The listing builds one solid part. Answer for the finished solid, in the listing's coordinates (mm). A direction names the side the tool comes from. Give positions to 0.01 mm unless a question says otherwise; leave off trailing zeros. Write each loop counter-clockwise with the first axis right and the second up, starting at its lowest first coordinate (ties: lowest second). Pieces come first, ordered by that corner, then holes. Notation, with made-up numbers: (-32, 39.25) - (22, 39.25) arc R31 ccw to (22, 74.25) - close; hole circle Ø11 at (32.25, -22.75). An arc over 180 degrees is marked (long way). Return JSON: item names as keys, results as strings.
from build123d import *
from OCP.BRepFilletAPI import BRepFilletAPI_MakeChamfer

# Parameters (mm, degrees)
SKETCH_1_W          = 44
SKETCH_1_H          = 24.5
EXTRUDE_1_DEPTH     = 20
SKETCH_2_W          = 57.5
SKETCH_2_H          = 24.5
EXTRUDE_2_DEPTH     = 3
CHAMFER_1_SIZE      = 3
CHAMFER_1_SIZE2     = 6
CHAMFER_2_SIZE      = 6
CHAMFER_2_SIZE2     = 3
CUT_EXTRUDE_1_DEPTH = 36.575623677
SKETCH_4_R          = 1.5
EXTRUDE_3_DEPTH     = 7
CUT_EXTRUDE_2_DEPTH = 20.5


with BuildPart() as part:
    # 草图1 → 凸台-拉伸1 (new body)
    with BuildSketch(Plane(origin=(0, 0, 0), x_dir=(1, 0, 0), z_dir=(0, 1, 0))):
        Rectangle(SKETCH_1_W, SKETCH_1_H)
    extrude(amount=EXTRUDE_1_DEPTH)

    # 草图2 → 凸台-拉伸2 (add)
    with BuildSketch(Plane.XZ):
        Rectangle(SKETCH_2_W, SKETCH_2_H)
    extrude(amount=-EXTRUDE_2_DEPTH)

    # 倒角1: one chamfer whose edges measure the first distance from different faces: ONE call of the kernel's chamfer builder (chamfer() names one face for all edges)
    chamfer_1_edges_1 = [part.edges().sort_by_distance(p)[0] for p in [
        (-28.75, 1.5, 12.25),
    ]]
    chamfer_1_side_1 = [part.faces().sort_by_distance(p)[0] for p in [
        (-28.75, 1.5, 0),
    ]]
    chamfer_1_edges_2 = [part.edges().sort_by_distance(p)[0] for p in [
        (28.75, 1.5, -12.25),
    ]]
    chamfer_1_side_2 = [part.faces().sort_by_distance(p)[0] for p in [
        (28.75, 1.5, 0),
    ]]
    chamfer_1 = BRepFilletAPI_MakeChamfer(part.part.solid().wrapped)
    for e in chamfer_1_edges_1:
        chamfer_1.Add(CHAMFER_1_SIZE, CHAMFER_1_SIZE2, e.wrapped, chamfer_1_side_1[0].wrapped)  # the first distance lies on this face
    for e in chamfer_1_edges_2:
        chamfer_1.Add(CHAMFER_1_SIZE, CHAMFER_1_SIZE2, e.wrapped, chamfer_1_side_2[0].wrapped)  # the first distance lies on this face
    add(Compound.cast(chamfer_1.Shape()), mode=Mode.REPLACE)

    # 倒角2: one chamfer whose edges measure the first distance from different faces: ONE call of the kernel's chamfer builder (chamfer() names one face for all edges)
    chamfer_2_edges_1 = [part.edges().sort_by_distance(p)[0] for p in [
        (-28.75, 1.5, -12.25),
    ]]
    chamfer_2_side_1 = [part.faces().sort_by_distance(p)[0] for p in [
        (-0.513573407, 9.788088643, -12.25),
    ]]
    chamfer_2_edges_2 = [part.edges().sort_by_distance(p)[0] for p in [
        (28.75, 1.5, 12.25),
    ]]
    chamfer_2_side_2 = [part.faces().sort_by_distance(p)[0] for p in [
        (0.513573407, 9.788088643, 12.25),
    ]]
    chamfer_2 = BRepFilletAPI_MakeChamfer(part.part.solid().wrapped)
    for e in chamfer_2_edges_1:
        chamfer_2.Add(CHAMFER_2_SIZE, CHAMFER_2_SIZE2, e.wrapped, chamfer_2_side_1[0].wrapped)  # the first distance lies on this face
    for e in chamfer_2_edges_2:
        chamfer_2.Add(CHAMFER_2_SIZE, CHAMFER_2_SIZE2, e.wrapped, chamfer_2_side_2[0].wrapped)  # the first distance lies on this face
    add(Compound.cast(chamfer_2.Shape()), mode=Mode.REPLACE)

    # 草图3 → 切除-拉伸1 (cut, through all)
    with BuildSketch(Plane(origin=(0, 3, 0), x_dir=(1, 0, 0), z_dir=(0, 1, 0))):
        with BuildLine():
            Line((-25.5, 2), (-28.75, 2))
            Line((-28.75, 2), (-28.75, -2))
            Line((-28.75, -2), (-25.5, -2))
            ThreePointArc((-25.5, -2), (-23.5, 0), (-25.5, 2))
        make_face()
        with BuildLine():
            Line((28.75, -2), (25.5, -2))
            ThreePointArc((25.5, -2), (23.5, 0), (25.5, 2))
            Line((25.5, 2), (28.75, 2))
            Line((28.75, 2), (28.75, -2))
        make_face()
    extrude(amount=-CUT_EXTRUDE_1_DEPTH, mode=Mode.SUBTRACT)

    # 草图4 → 凸台-拉伸3 (add)
    with BuildSketch(Plane.ZY.offset(22)):
        with Locations(Location((-6, 11.5, 0), (0, 0, 180))):
            Circle(SKETCH_4_R)
        with Locations(Location((6, 11.5, 0), (0, 0, 180))):
            Circle(SKETCH_4_R)
    extrude_3 = extrude(amount=EXTRUDE_3_DEPTH)

    # 镜向1: 凸台-拉伸3 across plane
    add(extrude_3.mirror(Plane.ZY))

    # 草图5 → 切除-拉伸2 (cut, symmetric)
    with BuildSketch(Plane(origin=(0, 0, 0), x_dir=(0, 0, -1), z_dir=(1, 0, 0))):
        Polygon((-12.25, 3), (-12.25, 0), (-12.15, 0), (-12.15, 3.1), (-12.15, 19.9), (12.15, 19.9), (12.15, 3.1), (12.15, 0), (12.25, 0), (12.25, 3), (12.25, 20), (-12.25, 20), align=None)
    extrude(amount=CUT_EXTRUDE_2_DEPTH, both=True, mode=Mode.SUBTRACT)


solid = part.part
Item 1: A cutting plane is placed at D-D on y = 11.5. Determine the outline of the cut face in (x, z), then the cut area to 3 significant figures.
Answer below:
{"outline": "(-29, -7.5) - (-22, -7.5) - (-22, -12.25) - (-20.5, -12.25) - (-20.5, -12.15) - (20.5, -12.15) - (20.5, -12.25) - (22, -12.25) - (22, -7.5) - (29, -7.5) - (29, -4.5) - (22, -4.5) - (22, 4.5) - (29, 4.5) - (29, 7.5) - (22, 7.5) - (22, 12.25) - (20.5, 12.25) - (20.5, 12.15) - (-20.5, 12.15) - (-20.5, 12.25) - (-22, 12.25) - (-22, 7.5) - (-29, 7.5) - (-29, 4.5) - (-22, 4.5) - (-22, -4.5) - (-29, -4.5) - close", "area": "1,150 mm²"}
Item 2: A cutting plane is placed at C-C on z = 0. Determine the outline of the cut face in (x, y).
Answer below:
{"outline": "(-23.5, 0) - (23.5, 0) - (23.5, 3) - (22, 3) - (22, 20) - (20.5, 20) - (20.5, 19.9) - (-20.5, 19.9) - (-20.5, 20) - (-22, 20) - (-22, 3) - (-23.5, 3) - close"}
Item 3: A cutting plane is placed at A-A on z = -6. Determine the outline of the cut face in (x, y), then the cut area to 3 significant figures.
Answer below:
{"outline": "(-29, 10) - (-22, 10) - (-22, 3) - (-28.75, 3) - (-28.75, 0) - (28.75, 0) - (28.75, 3) - (22, 3) - (22, 10) - (29, 10) - (29, 13) - (22, 13) - (22, 20) - (20.5, 20) - (20.5, 19.9) - (-20.5, 19.9) - (-20.5, 20) - (-22, 20) - (-22, 13) - (-29, 13) - close", "area": "958 mm²"}
Item 4: A cutting plane is placed at B-B on y = 16. Determine the outline of the cut face in (x, z).
Answer below:
{"outline": "(-22, -12.25) - (-20.5, -12.25) - (-20.5, -12.15) - (20.5, -12.15) - (20.5, -12.25) - (22, -12.25) - (22, 12.25) - (20.5, 12.25) - (20.5, 12.15) - (-20.5, 12.15) - (-20.5, 12.25) - (-22, 12.25) - close"}
Item 5: The mould has two halves that part along Y. Classify faces 1 (the face through (21, 20, 0)), 2 (the face through (23, 3, 0)), 3 (the face through (-27, 2, -2)): +Y half, -Y half, draft (parallel to the pull), parting line (faces both ways), or undercut.
Answer below:
{"face 1": "+Y half", "face 2": "undercut", "face 3": "draft"}
Item 6: Consider L1, parallel to Z at x = -5, y = 17.25; L2, parallel to Y at x = -17, z = -2; L3, parallel to X at y = 8, z = -7. Determine where each line is inside the solid, lowest interval first.
Answer below:
{"L1": "z = -12.15 to 12.15", "L2": "y = 0 to 19.9", "L3": "x = -22 to 22"}
Item 7: Flat-ended cylindrical pins translate along their axes: P1, Ø4, axis at x = -8.5, z = 7, coming from the +Y side; P2, Ø1, axis at x = 10.5, y = 5.5, coming from the +Z side; P3, Ø3.5, axis at x = -26.5, y = 1, coming from the -Z side. Find the tip coordinate at first contact, or state that the pin passes through.
Answer below:
{"P1": "stops at y = 19.9", "P2": "stops at z = 12.15", "P3": "stops at z = -11.25"}
Item 8: For faces 4 (the face through (28.75, 1, -6)), 5 (the face through (-28.75, 1, -6)), 6 (the face through (27, 2, 2)), 7 (the face through (0, 10, 12.15)), 8 (the face through (0, 19.9, 0)), determine the directions among +Z, -Z, +X, -X, +Y, -Y from which every point of the face is accessible in a straight line to the end or side of a thin tool.
Answer below:
{"face 4": "+Z, -Z, +X, -Y", "face 5": "+Z, -Z, -X, -Y", "face 6": "+X, +Y, -Y", "face 7": "+Z, +Y, -Y", "face 8": "+Z, -Z, +Y"}
